```python
from build123d import *

# Parameters (mm, degrees)
SKETCH_1_R          = 10
EXTRUDE_1_DEPTH     = 10
EXTRUDE_START       = -10
SKETCH_1_4_R        = 10
EXTRUDE_2_DEPTH     = 10
SKETCH_2_W          = 5
SKETCH_2_H          = 10
EXTRUDE_6_DEPTH     = 55
EXTRUDE_6_2_DEPTH   = 55
SKETCH_2_5_W        = 5
SKETCH_2_5_H        = 10
EXTRUDE_7_DEPTH     = 5
EXTRUDE_8_DEPTH     = 175
CUT_EXTRUDE_1_DEPTH = 175
SKETCH_7_W          = 10
SKETCH_7_H          = 10
CUT_EXTRUDE_2_DEPTH = 50
EXTRUDE_9_DEPTH     = 10
EXTRUDE_START_2     = 10
EXTRUDE_10_DEPTH    = 10


with BuildPart() as part:
    # Sketch 1 → Extrude 1 (new body)
    with BuildSketch(Plane.XY):
        Circle(SKETCH_1_R)
        with BuildLine():
            ThreePointArc((10, 0), (0, -10), (-10, 0))
            Line((-10, 0), (-10, -60))
            Line((-10, -60), (10, -60))
            Line((10, -60), (10, 0))
        make_face()
    extrude(amount=EXTRUDE_1_DEPTH)

    # Sketch 1_4 → Extrude 2 (add)
    with BuildSketch(Plane.XY.offset(EXTRUDE_START)):
        Circle(SKETCH_1_4_R)
    extrude(amount=EXTRUDE_2_DEPTH)



with BuildPart() as body_2:
    # Sketch 2 → Extrude 6 (new body)
    with BuildSketch(Plane.XZ.offset(60)):
        with Locations((-90, 5)):
            Rectangle(SKETCH_2_W, SKETCH_2_H)
    extrude(amount=EXTRUDE_6_DEPTH)


with BuildPart() as body_3:
    # Sketch 2 → Extrude 6 2 (new body)
    with BuildSketch(Plane.XZ.offset(60)):
        with Locations((90, 5)):
            Rectangle(SKETCH_2_W, SKETCH_2_H)
    extrude(amount=EXTRUDE_6_2_DEPTH)


with BuildPart() as part_1:
    add(part.part)

    add(body_2.part)  # Extrude 7 merges body 2

    add(body_3.part)  # Extrude 7 merges body 3
    # Sketch 2_5 → Extrude 7 (add)
    with BuildSketch(Plane.XZ.offset(60)):
        Polygon((-87.5, 0), (0, 0), (87.5, 0), (87.5, 10), (-87.5, 10), align=None)
        with Locations((-90, 5)):
            Rectangle(SKETCH_2_5_W, SKETCH_2_5_H)
        with Locations((90, 5)):
            Rectangle(SKETCH_2_5_W, SKETCH_2_5_H)
    extrude(amount=EXTRUDE_7_DEPTH)

    # Sketch 5 → Extrude 8 (add)
    with BuildSketch(Plane(origin=(-87.5, 0, 0), x_dir=(0, 0, -1), z_dir=(1, 0, 0))):
        with BuildLine():
            ThreePointArc((-8.535533906, -113.535533906), (-5, -115), (-1.464466094, -113.535533906))
            Line((-1.464466094, -113.535533906), (-5, -110))
            Line((-5, -110), (-8.535533906, -113.535533906))
        make_face()
        with BuildLine():
            Line((-5, -110), (-1.464466094, -113.535533906))
            ThreePointArc((-1.464466094, -113.535533906), (-0.380602337, -111.913417162), (0, -110))
            ThreePointArc((0, -110), (-0.380602337, -108.086582838), (-1.464466094, -106.464466094))
            Line((-1.464466094, -106.464466094), (-5, -110))
        make_face()
        with BuildLine():
            Line((-8.535533906, -113.535533906), (-5, -110))
            Line((-5, -110), (-8.535533906, -106.464466094))
            ThreePointArc((-8.535533906, -106.464466094), (-10, -110), (-8.535533906, -113.535533906))
        make_face()
        with BuildLine():
            Line((-8.535533906, -106.464466094), (-5, -110))
            Line((-5, -110), (-1.464466094, -106.464466094))
            ThreePointArc((-1.464466094, -106.464466094), (-3.086582829, -105.380602341), (-4.999999981, -105))
            ThreePointArc((-4.999999981, -105), (-6.913417153, -105.380602334), (-8.535533906, -106.464466094))
        make_face()
    extrude(amount=EXTRUDE_8_DEPTH)

    # Sketch 6 → Cut-Extrude 1 (cut)
    with BuildSketch(Plane(origin=(0, 0, -10), x_dir=(-1, 0, 0), z_dir=(0, 0, -1))):
        Polygon((0, -10), (-10, -10), (-10, 10), (10, 10), (10, -10), align=None)
    extrude(amount=-CUT_EXTRUDE_1_DEPTH, mode=Mode.SUBTRACT)

    # Sketch 7 → Cut-Extrude 2 (cut)
    with BuildSketch(Plane(origin=(0, -10, 0), x_dir=(1, 0, 0), z_dir=(0, 1, 0))):
        with Locations((5, -5)):
            Rectangle(SKETCH_7_W, SKETCH_7_H)
    extrude(amount=-CUT_EXTRUDE_2_DEPTH, mode=Mode.SUBTRACT)

    # Sketch 8 → Extrude 9 (add)
    with BuildSketch(Plane(origin=(0, 0, 0), x_dir=(0, 0, -1), z_dir=(1, 0, 0))):
        with BuildLine():
            ThreePointArc((5, 0), (-10, 8.660254038), (-10, -8.660254038))
            Line((-10, -8.660254038), (-10, 0))
            Line((-10, 0), (0, 0))
            Line((0, 0), (0, -8.660254038))
            ThreePointArc((0, -8.660254038), (3.660254038, -5), (5, 0))
        make_face()
        with BuildLine():
            Line((-10, 0), (-10, -8.660254038))
            ThreePointArc((-10, -8.660254038), (-7.588190451, -9.659258263), (-5, -10))
            ThreePointArc((-5, -10), (-2.411809549, -9.659258263), (0, -8.660254038))
            Line((0, -8.660254038), (0, 0))
            Line((0, 0), (-10, 0))
        make_face()
        with BuildLine():
            ThreePointArc((0, -8.660254038), (-2.411809549, -9.659258263), (-5, -10))
            Line((-5, -10), (0, -10))
            Line((0, -10), (0, -8.660254038))
        make_face()
        with BuildLine():
            Line((-10, -8.660254038), (-10, -10))
            Line((-10, -10), (-5, -10))
            ThreePointArc((-5, -10), (-7.588190451, -9.659258263), (-10, -8.660254038))
        make_face()
    extrude(amount=-EXTRUDE_9_DEPTH)

    # Sketch 8_3 → Extrude 10 (add)
    with BuildSketch(Plane(origin=(0, 0, 0), x_dir=(0, 0, -1), z_dir=(1, 0, 0)).offset(EXTRUDE_START_2)):
        with BuildLine():
            ThreePointArc((5, 0), (-10, 8.660254038), (-10, -8.660254038))
            Line((-10, -8.660254038), (-10, 0))
            Line((-10, 0), (0, 0))
            Line((0, 0), (0, -8.660254038))
            ThreePointArc((0, -8.660254038), (3.660254038, -5), (5, 0))
        make_face()
        with BuildLine():
            Line((-10, 0), (-10, -8.660254038))
            ThreePointArc((-10, -8.660254038), (-5, -10), (0, -8.660254038))
            Line((0, -8.660254038), (0, 0))
            Line((0, 0), (-10, 0))
        make_face()
    extrude(amount=-EXTRUDE_10_DEPTH)


solid = part_1.part
```
CAD build for the part. Positions are in the model's coordinates, mm. A direction names the side the tool comes from. Round coordinates to 2 decimals unless told otherwise and drop trailing zeros. Write each loop counter-clockwise with the first axis right and the second up, starting at its lowest first coordinate (ties: lowest second). Pieces come first, ordered by that corner, then holes.
Item 1: Drop flat-ended pins along their axis: pin 1 Ø3 at (y, z) = (-42.5, 7) entering from +X; pin 2 Ø6 at (y, z) = (-10.5, 9.5) entering from -X; pin 3 Ø10 at (x, y) = (46.5, -67) entering from +Z; pin 4 Ø10 at (x, z) = (7.5, 0.5) entering from +Y. Give the stop position or say it passes through.
Filled in:
pin 1: stops at x = 0
pin 2: stops at x = -10
pin 3: stops at z = 10
pin 4: stops at y = 10
Item 2: Band-saw the part on C-C on y = -57. Write the cut outline in (x, z), then the cut area to 3 significant figures.
Filled in:
outline: (-10, 0) - (0, 0) - (0, 10) - (-10, 10) - close
area: 100 mm2
Item 3: Mould opens along Y. For faces 5 (the flat face through (-1, -65, 5)), 6 (the flat face through (92.5, -87, 5)), 7 (the flat face through (90, -115, 5)), 8 (the flat face through (-52, -60, 5)) say: released by +Y, released by -Y, zero draft, split by the parting line, or undercut.
Filled in:
face 5: undercut
face 6: zero draft
face 7: released by -Y
face 8: released by +Y
Item 4: Band-saw the part on B-B on y = -78. Write the cut outline in (x, z), then the cut area to 3 significant figures.
Filled in:
outline: (-92.5, 0) - (-87.5, 0) - (-87.5, 10) - (-92.5, 10) - close; (87.5, 0) - (92.5, 0) - (92.5, 10) - (87.5, 10) - close
area: 100 mm2
Item 5: Band-saw the part on D-D on y = 0. Write the cut outline in (x, z).
Filled in:
outline: (-10, -5) - (10, -5) - (10, 15) - (-10, 15) - close
Item 6: Drill centre lines: L1, parallel to X at y = -99.5, z = 5.5; L2, parallel to Y at x = 5, z = 9.5; L3, parallel to Y at x = -70, z = 5.25. Where is each one in solid material? Low to high.
Filled in:
L1: x = -92.5 to -87.5, 87.5 to 92.5
L2: y = -112.18 to -107.82, -65 to -60, -8.93 to 8.93
L3: y = -114.99 to -105.01, -65 to -60
Item 7: Tool access for faces 1 (the flat face through (-87.5, -114, 9)), 2 (the cylindrical face through (0.14, 9.915, 6.302)), 3 (the flat face through (-87.5, -114, 1)), 4 (the flat face through (0, -62, 10)): list every direction of +Z, -Z, +X, -X, +Y, -Y with a clear straight run to the whole face (end or side of a thin tool).
Filled in:
face 1: +Z, -Y
face 2: +X
face 3: -Z, -Y
face 4: +Z, +X, -X, -Y
Item 8: Band-saw the part on A-A on x = -39. Write the cut outline in (y, z), then the cut area to 3 significant figures.
Filled in:
outline: circle Ø10 at (-110, 5); (-65, 0) - (-60, 0) - (-60, 10) - (-65, 10) - close
area: 129 mm2
